Part model, mm, in its own coordinate system. A direction names the side the tool comes from. Round coordinates to 2 decimals unless told otherwise and drop trailing zeros. Loops run counter-clockwise (first coordinate to the right, second up) from the corner with the lowest first, then second, coordinate; pieces in that order, holes last. Notation, with made-up numbers: (13.25, 11) -> (56.25, 11) arc R12 ccw to (56.25, 23) -> close; hole circle Ø11 at (-23.75, 76). An arc over 180 degrees is marked (long way). Use a Markdown table: item, result. Add a question column.
Item 1: Cut at B-B, the plane x = 0.5. List the corners of the cut face in (y, z), plus the area to 3 significant figures.
Item 2: Which spindle directions (+Z, -Z, +X, -X, +Y, -Y) get a long thin tool onto all of the face, cutting with end or side? Do faces 4 (the face through (7.341, 2.003, 9.369)), 5 (the face through (-4.5, -3.5, 8.2)). Say none if no direction does.
Item 3: Cut at A-A, the plane y = 0. List the corners of the cut face in (x, z).
Item 4: Two-plate mould, pull along Y, no slides. Class faces 1 (the face through (-4, 9.5, 5)), 2 (the face through (-7.386, 2.003, 9.369)), 3 (the face through (9, -0.1, 7.6)): pulls with the +Y half, pulls with the -Y half, needs draft (parallel to the pull), parting line crosses it, or undercut.
Item 5: Flat gauge pins, fed straight in: pin 1 (7.5 mm diameter, centred on x = 0, z = 10, fed in from +Y); pin 2 (8 mm diameter, centred on x = 3, y = -7, fed in from -Z). Where does each tip first touch, or does it go through?
Item 6: Cut at C-C, the plane y = 7.5. List the corners of the cut face in (x, z).
Item 7: Cut at D-D, the plane z = 4.5. List the corners of the cut face in (x, y).
Item 8: Probe line 1 (X direction, y = 5, z = 10); line 2 (Y direction, x = -6.95, z = 10); line 3 (Z direction, x = 0, y = 6). List the from-to ranges inside material, lowest first. Write a range as [from, to].
```python
from build123d import *

# Parameters (mm, degrees)
F0_W     = 18
F0_H     = 19
F1_DEPTH = 20
F3_R     = 6.1
F4_DEPTH = 13
F2_R     = 2.1
F5_DEPTH = 18
F6_R     = 3
F8_DEPTH = 25


with BuildPart() as f1:
    # F0 (on Top) → F1 (new body)
    with BuildSketch(Plane.XY):
        Rectangle(F0_W, F0_H)
    extrude(amount=F1_DEPTH)

    # F3 (on face) → F4 (cut)
    with BuildSketch(Plane(origin=(0, 9.5, 0), x_dir=(-1, 0, 0), z_dir=(0, 1, 0))):
        with Locations((0, 10)):
            Circle(F3_R)
    extrude(amount=-F4_DEPTH, mode=Mode.SUBTRACT)

    # F2 (on face) → F5 (cut)
    with BuildSketch(Plane.XZ.offset(9.5)):
        with Locations((0.5, 10)):
            Circle(F2_R)
    extrude(amount=-F5_DEPTH, mode=Mode.SUBTRACT)

    # F6
    f6_edges = [f1.edges().sort_by_distance(p)[0] for p in [
        (-1.6, -3.5, 10),
    ]]
    fillet(f6_edges, radius=F6_R)

    # F7 (on face) → F8 (cut)
    with BuildSketch(Plane(origin=(-9, 0, 0), x_dir=(0, -1, 0), z_dir=(-1, 0, 0))):
        with BuildLine():
            Line((-2.1, 10), (2.1, 10))
            ThreePointArc((2.1, 10), (0, 12.1), (-2.1, 10))
        make_face()
        with BuildLine():
            ThreePointArc((-2.1, 10), (0, 7.9), (2.1, 10))
            Line((2.1, 10), (-2.1, 10))
        make_face()
    extrude(amount=-F8_DEPTH, mode=Mode.SUBTRACT)


solid = f1.part
```
A:
| question | item | result |
|---|---|---|
| 1 | outline | (-9.5, 0) -> (9.5, 0) -> (9.5, 3.92) -> (-3.5, 3.92) -> (-3.5, 4.9) arc R3 ccw to (-6.5, 7.9) -> (-9.5, 7.9) -> close; (-9.5, 12.1) -> (-6.5, 12.1) arc R3 ccw to (-3.5, 15.1) -> (-3.5, 16.08) -> (9.5, 16.08) -> (9.5, 20) -> (-9.5, 20) -> close |
| 1 | area | 193 mm^2 |
| 2 | face 4 | +X, -X |
| 2 | face 5 | +Y |
| 3 | outline | (-9, 0) -> (9, 0) -> (9, 7.9) -> (5.73, 7.9) arc R6.1 cw to (-5.73, 7.9) -> (-9, 7.9) -> close; (-9, 12.1) -> (-5.73, 12.1) arc R6.1 cw to (5.73, 12.1) -> (9, 12.1) -> (9, 20) -> (-9, 20) -> close |
| 4 | face 1 | pulls with the +Y half |
| 4 | face 2 | undercut |
| 4 | face 3 | needs draft |
| 5 | pin 1 | stops at y = -3.62 |
| 5 | pin 2 | stops at z = 0 |
| 6 | outline | (-9, 0) -> (9, 0) -> (9, 20) -> (-9, 20) -> close; hole circle Ø12.2 at (0, 10) |
| 7 | outline | (-9, -9.5) -> (9, -9.5) -> (9, 9.5) -> (2.64, 9.5) -> (2.64, -3.5) -> (-2.64, -3.5) -> (-2.64, 9.5) -> (-9, 9.5) -> close |
| 8 | line 1 | x = [-9, -6.1], [6.1, 9] |
| 8 | line 2 | y = [-9.5, -2.1], [2.1, 9.5] |
| 8 | line 3 | z = [0, 3.9], [16.1, 20] |
